The listing builds one solid part. Answer for the finished solid, in the listing's coordinates (mm). A direction names the side the tool comes from. Give positions to 0.01 mm unless a question says otherwise; leave off trailing zeros. Loops run counter-clockwise (first coordinate to the right, second up) from the corner with the lowest first, then second, coordinate; pieces in that order, holes last. Notation, with made-up numbers: M 15.25,-10 L 43.25,-10 A33 cw 43.25,18 Z; hole C 80,-7 d10. An arc over 180 degrees is marked long. One line per item, written item: value. Start each with the question number.
Q1. The mould has two halves that part along Z. Classify faces 1 (the conical face through (44.187, 38.35, -57.996)), 2 (the cylindrical face through (-140.89, 34.42, -39.05)), 3 (the cylindrical face through (-21.77, 32.52, 86.92)), 4 (the flat face through (-19, 42.026, -31)): +Z half, -Z half, draft (parallel to the pull), parting line (faces both ways), or undercut.
Q2. For faces 5 (the cylindrical face through (-67.65, -49.37, 97.59)), 6 (the cylindrical face through (43.014, 32.516, -67.62)), determine the directions among +Z, -Z, +X, -X, +Y, -Y from which every point of the face is accessible in a straight line to the end or side of a thin tool.
Q3. Consider L1, parallel to Z at x = -17, y = 38; L2, parallel to Y at x = -11, z = 106; L3, parallel to X at y = 34, z = 66. Determine where each line is inside the solid, lowest interval first.
Q4. A cutting plane is placed at A-A, the plane y = -27. Determine the outline of the cut face in (x, z), and give its area (3 significant figures).
Q5. Flat-ended cylindrical pins translate along their axes: pin 1 (9 mm diameter, centred on x = -16.89, z = -89.46, fed in from +Y); pin 2 (10 mm diameter, centred on y = 30, z = -81.5, fed in from -X); pin 3 (12 mm diameter, centred on x = -119.5, y = -39.5, fed in from +Z); pin 4 (10 mm diameter, centred on x = -38.5, y = -22.5, fed in from -Z). Find the tip coordinate at first contact, or state that the pin passes through.
Q6. A cutting plane is placed at B-B, the plane z = 0. State how many separate pieces and enclosed holes the cut face has, and give its area (3 significant figures).
from build123d import *

# Parameters (mm, degrees)
CSK_FOR_M10_CROSS_COUNTERSUNK_HEAD_SCREW_D           = 11
CSK_FOR_M10_CROSS_COUNTERSUNK_HEAD_SCREW_CSINK_D     = 19
CSK_FOR_M10_CROSS_COUNTERSUNK_HEAD_SCREW_CSINK_ANGLE = 92
CIRPATTERN2_COUNT                                    = 8


with BuildPart() as part:
    # Sketch1 → Revolve2 (revolve)
    with BuildSketch(Plane.XY, mode=Mode.PRIVATE) as revolve2_sk:
        Polygon((13.106218235, 42.025554223), (113.106218235, 42.025554223), (113.106218235, 27.025554223), (53.106218235, 27.025554223), (53.106218235, -41.760408771), (93.106218235, -41.760408771), (93.106218235, -56.760408771), (13.106218235, -56.760408771), align=None)
    revolve(revolve2_sk.sketch.rotate(Axis((-16.893781765, 54.005560253, 0), (0, -1, 0)), 180), axis=Axis((-16.893781765, 54.005560253, 0), (0, -1, 0)))

    # CSK for M10 Cross Countersunk Head Screw1 (through all)
    with Locations(Plane(origin=(0, 42.025554223, 0), x_dir=(1, 0, 0), z_dir=(0, 1, 0))):
        with Locations((72.566522529, 0)):
            csk_for_m10_cross_countersunk_head_screw = CounterSinkHole(CSK_FOR_M10_CROSS_COUNTERSUNK_HEAD_SCREW_D / 2, CSK_FOR_M10_CROSS_COUNTERSUNK_HEAD_SCREW_CSINK_D / 2, counter_sink_angle=CSK_FOR_M10_CROSS_COUNTERSUNK_HEAD_SCREW_CSINK_ANGLE)

    # CirPattern2: CSK for M10 Cross Countersunk Head Screw1 ×8 about axis
    cirpattern2_axis = Axis((-16.893781765, 0, 0), (0, 1, 0))
    for i in range(1, CIRPATTERN2_COUNT):
        add(csk_for_m10_cross_countersunk_head_screw.rotate(cirpattern2_axis, i * 360 / CIRPATTERN2_COUNT), mode=Mode.SUBTRACT)


solid = part.part
Answer block:
1. face 1: undercut
1. face 2: parting line
1. face 3: undercut
1. face 4: draft
2. face 5: -Y
2. face 6: +Y, -Y
3. L1: -130 to -94.96, -83.96 to -30, 30 to 83.96, 94.96 to 130
3. L2: -56.76 to -41.76, 27.03 to 42.03
3. L3: -128.89 to -84.92, -75.38 to 41.6, 51.13 to 95.11
4. outline: C -16.89,0 d140; hole C -16.89,0 d60
4. area: 12,600 mm^2
5. pin 1: through
5. pin 2: x = -122
5. pin 3: z = 51.78
5. pin 4: z = -68
6. separate pieces: 6
6. enclosed holes: 0
6. area: 10,200 mm^2
